```python
from build123d import *

# Parameters (mm, degrees)
CROQUIS1_R              = 24.9
CROQUIS1_R_2            = 3.05
SALIENTE_EXTRUIR1_DEPTH = 2.5
CROQUIS2_R              = 30
SALIENTE_EXTRUIR2_DEPTH = 10.5
CROQUIS3_R              = 1.5
CORTAR_EXTRUIR1_DEPTH   = 44.706406853


with BuildPart() as part:
    # Croquis1 → Saliente-Extruir1 (new body)
    with BuildSketch(Plane(origin=(0, 0, 0), x_dir=(1, 0, 0), z_dir=(0, 1, 0))):
        with Locations(Location((0, 0, 0), (0, 0, 270))):
            Circle(CROQUIS1_R)
        with Locations(Location((0, 0, 0), (0, 0, 270))):
            Circle(CROQUIS1_R_2, mode=Mode.SUBTRACT)
    extrude(amount=SALIENTE_EXTRUIR1_DEPTH)

    # Croquis2 → Saliente-Extruir2 (add)
    with BuildSketch(Plane(origin=(0, 0, 0), x_dir=(1, 0, 0), z_dir=(0, 1, 0))):
        with Locations(Location((0, 0, 0), (0, 0, 270))):
            Circle(CROQUIS2_R)
        with BuildLine():
            Line((-4.135214626, 9.05), (4.135214626, 9.05))
            ThreePointArc((4.135214626, 9.05), (4.370264873, 9.021983221), (4.592144419, 8.939502762))
            ThreePointArc((4.592144419, 8.939502762), (10.05, 0), (4.592144419, -8.939502762))
            ThreePointArc((4.592144419, -8.939502762), (4.370264873, -9.021983221), (4.135214626, -9.05))
            Line((4.135214626, -9.05), (-4.135214626, -9.05))
            ThreePointArc((-4.135214626, -9.05), (-4.370264873, -9.021983221), (-4.592144419, -8.939502762))
            ThreePointArc((-4.592144419, -8.939502762), (-10.05, 0), (-4.592144419, 8.939502762))
            ThreePointArc((-4.592144419, 8.939502762), (-4.370264873, 9.021983221), (-4.135214626, 9.05))
        make_face(mode=Mode.SUBTRACT)
    extrude(amount=-SALIENTE_EXTRUIR2_DEPTH)

    # Croquis3 → Cortar-Extruir1 (cut, through all)
    with BuildSketch(Plane(origin=(0, 0, 0), x_dir=(1, 0, 0), z_dir=(0, 1, 0))):
        with Locations(Location((27.5, 0, 0), (0, 0, 270))):
            Circle(CROQUIS3_R)
        with Locations(Location((17.145969551, -21.500365768, 0), (0, 0, 270))):
            Circle(CROQUIS3_R)
        with Locations(Location((-6.119325684, -26.810517585, 0), (0, 0, 270))):
            Circle(CROQUIS3_R)
        with Locations(Location((-24.776643867, -11.931802826, 0), (0, 0, 270))):
            Circle(CROQUIS3_R)
        with Locations(Location((-24.776643867, 11.931802826, 0), (0, 0, 270))):
            Circle(CROQUIS3_R)
        with Locations(Location((-6.119325684, 26.810517585, 0), (0, 0, 270))):
            Circle(CROQUIS3_R)
        with Locations(Location((17.145969551, 21.500365768, 0), (0, 0, 270))):
            Circle(CROQUIS3_R)
    extrude(amount=-CORTAR_EXTRUIR1_DEPTH, mode=Mode.SUBTRACT)


solid = part.part
```
CAD build for the part. Positions are in the model's coordinates, mm. A direction names the side the tool comes from. Round coordinates to 2 decimals unless told otherwise and drop trailing zeros. Loops run counter-clockwise (first coordinate to the right, second up) from the corner with the lowest first, then second, coordinate; pieces in that order, holes last. Notation, with made-up numbers: M 84.5,-9.5 L 125.5,-9.5 A27 cw 125.5,27.5 Z; hole C -1,24 d5. An arc over 180 degrees is marked long. Use a Markdown table: item, result. Add a question column.
(1) Cut at A-A (z = 0). Give the cut face in (x, y).
(2) Which spindle directions (+Z, -Z, +X, -X, +Y, -Y) get a long thin tool onto all of the face, cutting with end or side? Do faces 4 (the face through (0, -5, -9.05)), 5 (the face through (-13, -10.5, 0)), 6 (the face through (-15.15, 1.23, -19.76)). Say none if no direction does.
(3) Flat gauge pins, fed straight in: pin 1 (4 mm diameter, centred on x = 3.5, y = -2, fed in from +Z); pin 2 (6.5 mm diameter, centred on x = 0.5, y = -4.5, fed in from -Z); pin 3 (5 mm diameter, centred on x = 0, z = 0, fed in from -Y); pin 4 (3.5 mm diameter, centred on x = -6.12, z = -26.81, fed in from +Y). Where does each tip first touch, or does it go through?
(4) Cut at C-C (y = -5.25). State how many separate pieces and enclosed holes the cut face has, and give its area (3 significant figures).
(5) Cut at D-D (z = 17.5). Give the cut face in (x, y), and give its area (3 significant figures).
(6) Pull direction X, two halves, no side cores. Call faces 1 (the face through (0, 0, -4)), 2 (the face through (1.32, -5.18, -29.97)), 3 (the face through (0, 2.5, 5)): +X half, -X half, draft (parallel to the pull), parting line (faces both ways), or undercut.
(7) Drill centre lines: line 1 (X direction, y = 1.55, z = 0); line 2 (Z direction, x = 0.5, y = -6); line 3 (X direction, y = -5.5, z = 27.5). Where is each one in solid material? Low to high.
(8) Cut at B-B (x = 0). Give the cut face in (y, z).
Geometry says:
| question | item | result |
|---|---|---|
| 1 | outline | M -30,-10.5 L -10.05,-10.5 L -10.05,0 L -3.05,0 L -3.05,2.5 L -24.9,2.5 L -24.9,0 L -30,0 Z; M 3.05,0 L 10.05,0 L 10.05,-10.5 L 26,-10.5 L 26,0 L 24.9,0 L 24.9,2.5 L 3.05,2.5 Z; M 29,-10.5 L 30,-10.5 L 30,0 L 29,0 Z |
| 2 | face 4 | -Y |
| 2 | face 5 | +Z, -Z, +X, -X, -Y |
| 2 | face 6 | +Y |
| 3 | pin 1 | stops at z = 29.96 |
| 3 | pin 2 | stops at z = -30 |
| 3 | pin 3 | passes through |
| 3 | pin 4 | stops at y = 0 |
| 4 | separate pieces | 1 |
| 4 | enclosed holes | 8 |
| 4 | area | 2,470 mm² |
| 5 | outline | M -24.37,-10.5 L 24.37,-10.5 L 24.37,0 L 17.71,0 L 17.71,2.5 L -17.71,2.5 L -17.71,0 L -24.37,0 Z |
| 5 | area | 600 mm² |
| 6 | face 1 | undercut |
| 6 | face 2 | parting line |
| 6 | face 3 | draft |
| 7 | line 1 | x = -24.9 to -3.05, 3.05 to 24.9 |
| 7 | line 2 | z = -30 to -9.05, 9.05 to 30 |
| 7 | line 3 | x = -11.99 to -7.45, -4.79 to 11.99 |
| 8 | outline | M -10.5,-30 L 0,-30 L 0,-24.9 L 2.5,-24.9 L 2.5,-3.05 L 0,-3.05 L 0,-9.05 L -10.5,-9.05 Z; M -10.5,9.05 L 0,9.05 L 0,3.05 L 2.5,3.05 L 2.5,24.9 L 0,24.9 L 0,30 L -10.5,30 Z |
